Design review of the part built by this model. Coordinates are the model's own, in mm. Give positions to 0.01 mm unless a question says otherwise; leave off trailing zeros. Write each loop counter-clockwise with the first axis right and the second up, starting at its lowest first coordinate (ties: lowest second). Pieces come first, ordered by that corner, then holes. Notation, with made-up numbers: (-8.5, 74) -> (11.5, 74) arc R21 ccw to (11.5, 111) -> close; hole circle Ø11 at (-5.5, 46). An arc over 180 degrees is marked (long way). Answer as a JSON object with one key per item and string values.
```python
from build123d import *

# Parameters (mm, degrees)
SKETCH1_W                      = 80
SKETCH1_H                      = 42
BOSS_EXTRUDE1_DEPTH            = 42
FILLET1_R                      = 4
CHAMFER1_SIZE                  = 0.5
CBORE_FOR_M4_SHCS1_D           = 4.5
CBORE_FOR_M4_SHCS1_CBORE_D     = 8
CBORE_FOR_M4_SHCS1_CBORE_DEPTH = 4
SKETCH5_R                      = 12.5
CUT_EXTRUDE2_DEPTH             = 62.684682053
CHAMFER2_SIZE                  = 0.5
CHAMFER3_SIZE                  = 0.3


with BuildPart() as part:
    # Sketch1 → Boss-Extrude1 (new body)
    with BuildSketch(Plane.XY):
        Rectangle(SKETCH1_W, SKETCH1_H)
    extrude(amount=BOSS_EXTRUDE1_DEPTH)

    # Fillet1
    fillet1_edges = [part.edges().sort_by_distance(p)[0] for p in [
        (40, -21, 21),
        (-40, -21, 21),
        (-40, 21, 21),
        (40, 21, 21),
    ]]
    fillet(fillet1_edges, radius=FILLET1_R)

    # Chamfer1
    chamfer1_edges = [part.edges().sort_by_distance(p)[0] for p in [
        (40, 0, 0),
        (40, 0, 42),
        (0, -21, 0),
        (-40, 0, 0),
        (0, 21, 0),
        (-38.828427125, 19.828427125, 0),
        (38.828427125, 19.828427125, 0),
        (-38.828427125, -19.828427125, 0),
        (38.828427125, -19.828427125, 0),
        (0, -21, 42),
        (0, 21, 42),
        (-40, 0, 42),
        (-38.828427125, 19.828427125, 42),
        (38.828427125, 19.828427125, 42),
        (-38.828427125, -19.828427125, 42),
        (38.828427125, -19.828427125, 42),
    ]]
    chamfer(chamfer1_edges, length=CHAMFER1_SIZE)

    # CBORE for M4 SHCS1 (through all)
    with Locations(Plane.XY.offset(42)):
        with Locations((-30, 10), (30, 10), (30, -10), (-30, -10)):
            CounterBoreHole(CBORE_FOR_M4_SHCS1_D / 2, CBORE_FOR_M4_SHCS1_CBORE_D / 2, CBORE_FOR_M4_SHCS1_CBORE_DEPTH)

    # Sketch5 → Cut-Extrude2 (cut, through all)
    with BuildSketch(Plane(origin=(0, 0, 0), x_dir=(-1, 0, 0), z_dir=(0, 0, -1))):
        Circle(SKETCH5_R)
    extrude(amount=-CUT_EXTRUDE2_DEPTH, mode=Mode.SUBTRACT)

    # Chamfer2
    chamfer2_edges = [part.edges().sort_by_distance(p)[0] for p in [
        (12.5, 0, 42),
        (12.5, 0, 0),
    ]]
    chamfer(chamfer2_edges, length=CHAMFER2_SIZE)

    # Chamfer3
    chamfer3_edges = [part.edges().sort_by_distance(p)[0] for p in [
        (26, 10, 42),
        (32.25, 10, 0),
        (32.25, 10, 38),
        (-34, 10, 42),
        (-27.75, 10, 0),
        (-27.75, 10, 38),
        (-34, -10, 42),
        (-27.75, -10, 0),
        (-27.75, -10, 38),
        (26, -10, 42),
        (32.25, -10, 0),
        (32.25, -10, 38),
    ]]
    chamfer(chamfer3_edges, length=CHAMFER3_SIZE)


solid = part.part
```
(1) The part is to be moulded in two halves that separate along Y. For faces 1 (the flat face through (-1, -21, 21)), 2 (the conical face through (-38.55, 19.6, 41.86)), 3 (the flat face through (33, -10, 38)), 4 (the flat face through (-9.3, 9.4, 0)), say which applies: +Y half, -Y half, draft (parallel to the pull), parting line (faces both ways), or undercut.
Here are the results:
{"face 1": "-Y half", "face 2": "+Y half", "face 3": "undercut", "face 4": "draft"}
(2) We need section A-A, the plane x = 0. State the section outline as (y, z) points.
Here are the results:
{"outline": "(-21, 0.5) -> (-20.5, 0) -> (-13, 0) -> (-12.5, 0.5) -> (-12.5, 41.5) -> (-13, 42) -> (-20.5, 42) -> (-21, 41.5) -> close; (12.5, 0.5) -> (13, 0) -> (20.5, 0) -> (21, 0.5) -> (21, 41.5) -> (20.5, 42) -> (13, 42) -> (12.5, 41.5) -> close"}
(3) We need section C-C, the plane x = 30. Give the number of separate pieces and of enclosed holes in the cut face, then the cut area to 3 significant figures.
Here are the results:
{"separate pieces": "3", "enclosed holes": "0", "area": "1,360 mm²"}
(4) For line 1 along Y through (x, z) = (30, 11.5); line 2 along Y through (x, z) = (-30, 40.65); line 3 along X through (y, z) = (8.5, 11), list the stretches that pass through material, from the lowest coordinate up.
Here are the results:
{"line 1": "y = -21 to -12.25, -7.75 to 7.75, 12.25 to 21", "line 2": "y = -21 to -14, -6 to 6, 14 to 21", "line 3": "x = -40 to -31.68, -28.32 to -9.17, 9.17 to 28.32, 31.68 to 40"}
(5) We need section B-B, the plane z = 26. State the section outline as (x, y) points.
Here are the results:
{"outline": "(-40, -17) arc R4 ccw to (-36, -21) -> (36, -21) arc R4 ccw to (40, -17) -> (40, 17) arc R4 ccw to (36, 21) -> (-36, 21) arc R4 ccw to (-40, 17) -> close; hole circle Ø4.5 at (-30, -10); hole circle Ø4.5 at (-30, 10); hole circle Ø25 at (0, 0); hole circle Ø4.5 at (30, -10); hole circle Ø4.5 at (30, 10)"}
(6) Clearance check with flat-ended pins moving along their axes: pin 1 (4 mm diameter, centred on x = -30.5, y = -11, fed in from +Z); pin 2 (3.5 mm diameter, centred on x = -30, y = 10, fed in from +Z). State where each tip first meets the part, or that it passes through.
Here are the results:
{"pin 1": "stops at z = 38", "pin 2": "passes through"}
